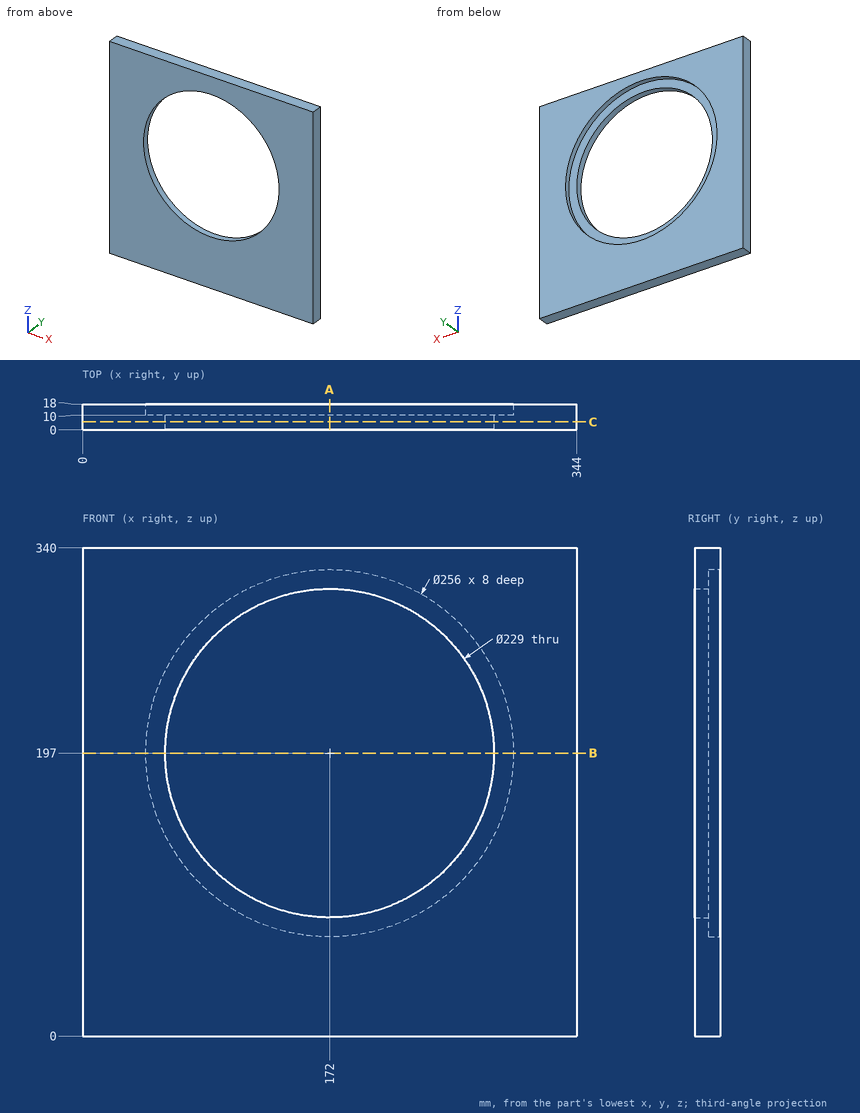
Here's the drawing with two shaded views (mm, measured from the low corner). I have some questions. Coordinates: 2 decimals unless noted, no trailing zeros. Write each loop counter-clockwise with the first axis right and the second up, starting at its lowest first coordinate (ties: lowest second). Pieces come first, ordered by that corner, then holes. Notation, with made-up numbers: M -12.75,-12.5 L 9.25,-12.5 A5 ccw 9.25,-7.5 Z; hole C -5.5,71 d8. An arc over 180 degrees is marked long. Use one line per item in the form item = value.
Q1. For P1, Ø5, axis at y = 2, z = 289, coming from the -X side; P2, Ø12, axis at x = 287, z = 195, coming from the +Y side, each with a flat end and sliding along its axis, tell me the tip position at first contact or that it passes through.
Model answer:
P1 = 0
P2 = 10
Q2. I need wall thicknesses on line 1 along Z through (x, y) = (172, 2.25); line 2 along X through (y, z) = (6, 197); line 3 along Z through (x, y) = (172, 14.5). Which ranges of each line are inside material? Lowest first, please. Write a range as from..to.
Model answer:
line_1 = 0..82.5, 311.5..340
line_2 = 0..57.5, 286.5..344
line_3 = 0..69, 325..340
Q3. If we section it at A-A (x = 172): Write out the boundary of the cut face in (y, z).
Model answer:
outline = M 0,0 L 18,0 L 18,69 L 10,69 L 10,82.5 L 0,82.5 Z; M 0,311.5 L 10,311.5 L 10,325 L 18,325 L 18,340 L 0,340 Z
Q4. If we section it at C-C (y = 5.5): Write out the boundary of the cut face in (x, z).
Model answer:
outline = M 0,0 L 344,0 L 344,340 L 0,340 Z; hole C 172,197 d229
Q5. If we section it at B-B (z = 197): Write out the boundary of the cut face in (x, y).
Model answer:
outline = M 0,0 L 57.5,0 L 57.5,10 L 44,10 L 44,18 L 0,18 Z; M 286.5,0 L 344,0 L 344,18 L 300,18 L 300,10 L 286.5,10 Z
